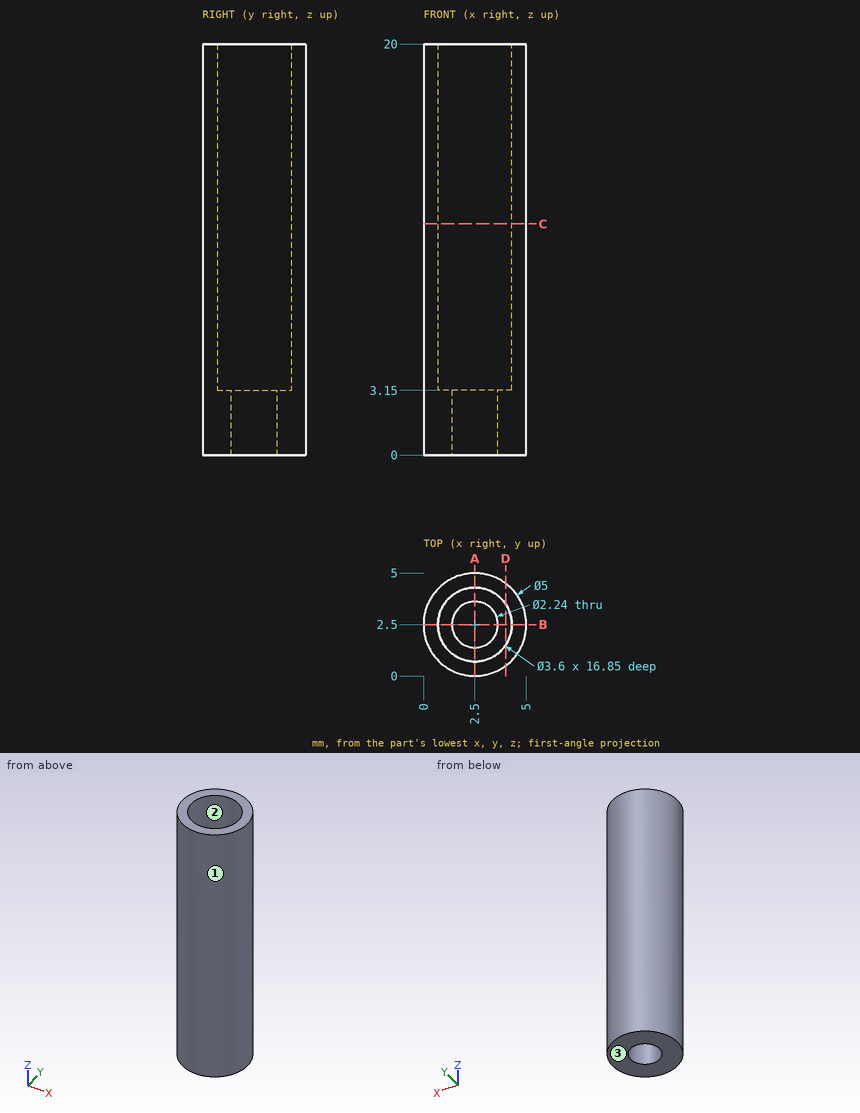
Source: three-view drawing plus pictorial views. Frame: mm from the lowest corner of the part. Round coordinates to 2 decimals unless told otherwise and drop trailing zeros. Order: outer loops, then holes, each group sorted by start corner. A loop starts at its lowest first (then second) coordinate and runs counter-clockwise, first axis right, second up. Notation, with made-up numbers: (89, 69) -> (109, 69) arc R19 ccw to (109, 101) -> close; hole circle Ø10 at (21.5, 51). An arc over 180 degrees is marked (long way). Use one line per item in the form item = value. Start each with the question number.
1. Pin query (flat end, axial travel): pin 1 Ø1 at (x, z) = (0.5, 17.5) entering from +Y; pin 2 Ø3 at (x, z) = (4.5, 2.5) entering from +Y. Return the tip coordinate at first contact, or that it passes through.
2. Cut plane A-A (x = 2.5). Return the cut outline in (y, z), then the cut area to 3 significant figures.
3. Line query: probe 1 along Y at (x, z) = (2.5, 7.25); probe 2 along Y at (x, z) = (2.5, 1.4); probe 3 along Z at (x, y) = (3.9, 3.2). Output: solid intervals per line, ascending.
4. Cut plane C-C (z = 11.25). Return the cut outline in (x, y).
5. Cut plane D-D (x = 4). Return the cut outline in (y, z), then the cut area to 3 significant figures.
6. Draft query along X for the marked faces 1, 2 and 3. Return one class per face: pulls with the +X half, pulls with the -X half, needs draft (parallel to the pull), parting line crosses it, or undercut.
Solution:
q1.pin_1 = 4.5
q1.pin_2 = 4.95
q2.outline = (0, 0) -> (1.38, 0) -> (1.38, 3.15) -> (0.7, 3.15) -> (0.7, 20) -> (0, 20) -> close; (3.62, 0) -> (5, 0) -> (5, 20) -> (4.3, 20) -> (4.3, 3.15) -> (3.62, 3.15) -> close
q2.area = 32.3 mm^2
q3.probe_1 = 0 to 0.7, 4.3 to 5
q3.probe_2 = 0 to 1.38, 3.62 to 5
q3.probe_3 = 0 to 3.15
q4.outline = circle Ø5 at (2.5, 2.5); hole circle Ø3.6 at (2.5, 2.5)
q5.outline = (0.5, 0) -> (4.5, 0) -> (4.5, 20) -> (3.49, 20) -> (3.49, 3.15) -> (1.51, 3.15) -> (1.51, 20) -> (0.5, 20) -> close
q5.area = 46.5 mm^2
q6.face_1 = parting line crosses it
q6.face_2 = undercut
q6.face_3 = needs draft
